from build123d import *

# Parameters (mm, degrees)
F0_R     = 11.1125
F1_DEPTH = 87.3125
F2_R     = 7.9375
F3_DEPTH = 127
F4_W     = 41.7499989271
F4_H     = 12.747396715
F5_DEPTH = 127


with BuildPart() as f1:
    # F0 (on Front) → F1 (new body, symmetric)
    with BuildSketch(Plane.XZ):
        Circle(F0_R)
    extrude(amount=F1_DEPTH, both=True)

    # F2 (on Front) → F3 (cut, symmetric)
    with BuildSketch(Plane.XZ):
        Circle(F2_R)
    extrude(amount=F3_DEPTH, both=True, mode=Mode.SUBTRACT)

    # F4 (on Front) → F5 (cut, symmetric)
    with BuildSketch(Plane.XZ):
        with Locations((-0.1250002533, 6.3736983575)):
            Rectangle(F4_W, F4_H)
    extrude(amount=F5_DEPTH, both=True, mode=Mode.SUBTRACT)


solid = f1.part
The listing builds one solid part. Answer for the finished solid, in the listing's coordinates (mm). Round coordinates to 2 decimals unless told otherwise and drop trailing zeros. Order: outer loops, then holes, each group sorted by start corner. A loop starts at its lowest first (then second) coordinate and runs counter-clockwise, first axis right, second up. Notation, with made-up numbers: M -18,85 L 22,85 A24 ccw 22,107 Z; hole C 54.25,-6.75 d11. An arc over 180 degrees is marked long. Answer in a Markdown table with one row per item. Add a question column.
1) Flat-ended cylindrical pins translate along their axes: pin 1 Ø8 at (x, y) = (0.5, -35.5) entering from -Z; pin 2 Ø3 at (x, y) = (-8.5, -34) entering from -Z; pin 3 Ø5 at (x, y) = (-5.5, -9) entering from -Z; pin 4 Ø6 at (x, y) = (6.5, 15) entering from -Z. Find the tip coordinate at first contact, or state that the pin passes through.
2) The part is cut by section A-A on z = -4.5. Determine the outline of the cut face in (x, y).
3) The part is cut by section C-C on y = 3. Determine the outline of the cut face in (x, z) (1 decimal), plus the area to 3 significant figures.
4) Consider line 1 along Z through (x, y) = (0.25, 38); line 2 along X through (y, z) = (-53.5, -4.5); line 3 along X through (y, z) = (-37, -4.25). Determine where each line is inside the solid, lowest interval first. Write a range as from..to.
5) The part is cut by section B-B on x = 0. Determine the outline of the cut face in (y, z), plus the area to 3 significant figures.
Findings below:
| question | item | result |
|---|---|---|
| 1 | pin 1 | stops at z = -11.11 |
| 1 | pin 2 | stops at z = -8.63 |
| 1 | pin 3 | stops at z = -10.7 |
| 1 | pin 4 | stops at z = -10.55 |
| 2 | outline | M -10.16,-87.31 L -6.54,-87.31 L -6.54,87.31 L -10.16,87.31 Z; M 6.54,-87.31 L 10.16,-87.31 L 10.16,87.31 L 6.54,87.31 Z |
| 3 | outline | M -11.1,0 A11.1 ccw 11.1,0 L 7.9,0 A7.9 cw -7.9,0 Z |
| 3 | area | 95.0 mm² |
| 4 | line 1 | z = -11.11..-7.93 |
| 4 | line 2 | x = -10.16..-6.54, 6.54..10.16 |
| 4 | line 3 | x = -10.27..-6.7, 6.7..10.27 |
| 5 | outline | M -87.31,-11.11 L 87.31,-11.11 L 87.31,-7.94 L -87.31,-7.94 Z |
| 5 | area | 554 mm² |
